Input: part model. Units: mm. Frame: model coordinates. A direction names the side the tool comes from. Give positions to 0.01 mm unless a question says otherwise; leave off trailing zeros. Loops run counter-clockwise (first coordinate to the right, second up) from the corner with the lowest first, then second, coordinate; pieces in that order, holes last. Notation, with made-up numbers: M 89,43 L 132,43 A28 cw 132,75 Z; hole C -2,78 d1. An arc over 180 degrees is marked long. Use CSV: the item, a comma, the result in double quotes. Start each with the question number.
from build123d import *

# Parameters (mm, degrees)
HEAD_DEPTH = 4.7
SKBODY_R   = 2.5
BODY_DEPTH = 20


with BuildPart() as part:
    # skHead → Head (new body)
    with BuildSketch(Plane(origin=(0, 0, 0), x_dir=(1, 0, 0), z_dir=(0, 1, 0))):
        Polygon((4.618802154, 0), (2.309401077, 4), (-2.309401077, 4), (-4.618802154, 0), (-2.309401077, -4), (2.309401077, -4), align=None)
    extrude(amount=HEAD_DEPTH)

    # skBody → Body (add)
    with BuildSketch(Plane(origin=(0, 0, 0), x_dir=(1, 0, 0), z_dir=(0, 1, 0))):
        with Locations(Location((0, 0, 0), (0, 0, 270))):
            Circle(SKBODY_R)
    extrude(amount=-BODY_DEPTH)


solid = part.part
Item 1: Section C-C (z = -0.75). Output: boundary loops of the cut face in (x, y).
Item 2: Section D-D (y = -14.5). Output: boundary loops of the cut face in (x, z).
Item 3: First-contact query: pin 1 Ø3 at (y, z) = (-6.5, 2.5) entering from +X; pin 2 Ø2 at (x, z) = (-3.5, 0.5) entering from -Y; pin 3 Ø1 at (x, y) = (-3.5, -1) entering from -Z; pin 4 Ø1.5 at (y, z) = (-2.5, 3) entering from -X. Flat tips, straight axial feed; report the tip coordinate or a pass-through.
Item 4: Section A-A (x = -1.5). Output: boundary loops of the cut face in (y, z).
Item 5: Section B-B (y = 0.25). Output: boundary loops of the cut face in (x, z).
Item 6: Material intervals for line 1 (Y direction, x = -0.5, z = -3.5); line 2 (X direction, y = -0.5, z = 0); line 3 (X direction, y = -17.5, z = 2), sorted ascending.
Item 7: Set-up query: faces 1 (the cylindrical face through (-2.44, -9.86, -0.54)), 2 (the flat face through (0, 2, -4)). Return all of +Z, -Z, +X, -X, +Y, -Y with unobstructed straight access to the full face (end or side cutting, diameter ignored); none if empty.
Recorded:
1,outline,"M -4.19,0 L -2.38,0 L -2.38,-20 L 2.38,-20 L 2.38,0 L 4.19,0 L 4.19,4.7 L -4.19,4.7 Z"
2,outline,"C 0,0 d5"
3,pin 1,"x = 2.29"
3,pin 2,"y = 0"
3,pin 3,"through"
3,pin 4,"x = -1.09"
4,outline,"M -20,-2 L 0,-2 L 0,-4 L 4.7,-4 L 4.7,4 L 0,4 L 0,2 L -20,2 Z"
5,outline,"M -4.62,0 L -2.31,-4 L 2.31,-4 L 4.62,0 L 2.31,4 L -2.31,4 Z"
6,line 1,"0 to 4.7"
6,line 2,"-2.5 to 2.5"
6,line 3,"-1.5 to 1.5"
7,face 1,"-Y"
7,face 2,"-Z, +X, -X, +Y, -Y"
